Geometry check sheet. Reference: the model listing, model coordinates, mm. A direction names the side the tool comes from. Round coordinates to 2 decimals unless told otherwise and drop trailing zeros. Write each loop counter-clockwise with the first axis right and the second up, starting at its lowest first coordinate (ties: lowest second). Pieces come first, ordered by that corner, then holes. Notation, with made-up numbers: (13.5, 71) - (36.5, 71) arc R8 cw to (36.5, 81) - close; hole circle Ø9 at (71.5, -22). An arc over 180 degrees is marked (long way). One line per question, with ' | ' between items. Start each with the question number.
from build123d import *

# Parameters (mm, degrees)
EXTRUDE_1_DEPTH           = 7
SKETCH_6_R                = 7
EXTRUDE_5_DEPTH           = 13
SKETCH_8_R                = 2
CUT_EXTRUDE_2_DEPTH       = 30
SKETCH_9_R                = 5
CUT_EXTRUDE_3_DEPTH       = 2.65
CUT_EXTRUDE_START         = -2.65
SKETCH_10_R               = 5
CUT_EXTRUDE_4_DEPTH       = 2.65
HOLE_WIZARD_2_D           = 3.5
HOLE_WIZARD_2_DEPTH       = 20
HOLE_WIZARD_2_CBORE_D     = 6.5
HOLE_WIZARD_2_CBORE_DEPTH = 3.1
HOLE_WIZARD_2_TIP         = 1.051506083


with BuildPart() as part:
    # 草图1 → 凸台-拉伸1 (new body)
    with BuildSketch(Plane(origin=(0, 0, 0), x_dir=(1, 0, 0), z_dir=(0, 1, 0))):
        with BuildLine():
            Line((9.486832981, -13.5), (-9.486832981, -13.5))
            ThreePointArc((-9.486832981, -13.5), (-11.66726189, -11.66726189), (-13.5, -9.486832981))
            Line((-13.5, -9.486832981), (-13.5, 9.486832981))
            ThreePointArc((-13.5, 9.486832981), (-11.66726189, 11.66726189), (-9.486832981, 13.5))
            Line((-9.486832981, 13.5), (9.486832981, 13.5))
            ThreePointArc((9.486832981, 13.5), (11.66726189, 11.66726189), (13.5, 9.486832981))
            Line((13.5, 9.486832981), (13.5, -9.486832981))
            ThreePointArc((13.5, -9.486832981), (11.66726189, -11.66726189), (9.486832981, -13.5))
        make_face()
    extrude(amount=EXTRUDE_1_DEPTH)

    # 草图6 → 凸台-拉伸5 (add)
    with BuildSketch(Plane(origin=(0, 7, 0), x_dir=(1, 0, 0), z_dir=(0, 1, 0))):
        with Locations(Location((0, 0, 0), (0, 0, 90))):
            Circle(SKETCH_6_R)
    extrude(amount=EXTRUDE_5_DEPTH)

    # 草图8 → 切除-拉伸2 (cut)
    with BuildSketch(Plane(origin=(0, 20, 0), x_dir=(1, 0, 0), z_dir=(0, 1, 0))):
        with Locations(Location((0, 0, 0), (0, 0, 270))):
            Circle(SKETCH_8_R)
    extrude(amount=-CUT_EXTRUDE_2_DEPTH, mode=Mode.SUBTRACT)

    # 草图9 → 切除-拉伸3 (cut)
    with BuildSketch(Plane(origin=(0, 20, 0), x_dir=(1, 0, 0), z_dir=(0, 1, 0))):
        with Locations(Location((0, 0, 0), (0, 0, 270))):
            Circle(SKETCH_9_R)
    extrude(amount=-CUT_EXTRUDE_3_DEPTH, mode=Mode.SUBTRACT)

    # 草图10 → 切除-拉伸4 (cut)
    with BuildSketch(Plane.XZ.offset(CUT_EXTRUDE_START)):
        with Locations(Location((0, 0, 0), (0, 0, 90))):
            Circle(SKETCH_10_R)
    extrude(amount=CUT_EXTRUDE_4_DEPTH, mode=Mode.SUBTRACT)

    # 孔2
    with Locations(Plane(origin=(0, 0, 0), x_dir=(-1, 0, 0), z_dir=(0, -1, 0))):
        with Locations((-8.209852454, 8.492066132), (8.626364404, 8.339687642), (8.471576116, -8.762786544), (-8.626364404, -8.339687642)):
            CounterBoreHole(HOLE_WIZARD_2_D / 2, HOLE_WIZARD_2_CBORE_D / 2, HOLE_WIZARD_2_CBORE_DEPTH, depth=HOLE_WIZARD_2_DEPTH)
            with Locations((0, 0, -(HOLE_WIZARD_2_DEPTH + HOLE_WIZARD_2_TIP / 2))):  # 118° drill point
                Cone(0, HOLE_WIZARD_2_D / 2, HOLE_WIZARD_2_TIP, mode=Mode.SUBTRACT)


solid = part.part
Q1. Section check D-D, the plane y = 1.5. Record the cut outline in (x, z), then the cut area to 3 significant figures.
Q2. Go/stop test with flat-tipped pins: P1, Ø3, axis at x = 1, z = 0, coming from the -Y side; P2, Ø6.5, axis at x = 0, z = 0, coming from the +Y side; P3, Ø4, axis at x = 8.21, z = -8.49, coming from the -Y side. Record where each tip stops, or that it passes through.
Q3. Section check C-C, the plane x = 9. Record the cut outline in (y, z).
Q4. Draft check along X on faces 1 (the flat face through (-0.1, 2.65, 2.2)), 2 (the cylindrical face through (11.639, 3.451, -11.695)), 3 (the flat face through (0, 0, -6)). Enter one of: pulls with the +X half, pulls with the -X half, needs draft (parallel to the pull), parting line crosses it, or undercut.
Q5. Set-up check for faces 4 (the cylindrical face through (6.834, 13.409, 1.517)), 5 (the flat face through (-10, 3.1, 10)), 6 (the flat face through (0, 3, 13.5)): record each of +Z, -Z, +X, -X, +Y, -Y from which the full face is reachable in a straight line by a thin tool's end or side.
Q6. Section check A-A, the plane z = 0. Record the cut outline in (x, y).
Q7. Section check B-B, the plane x = 0. Record the cut outline in (y, z), then the cut area to 3 significant figures.
Q8. Thickness scan on line 1 (Z direction, x = 11, y = 2.25); line 2 (Z direction, x = 8.5, y = 3.25); line 3 (X direction, y = 0.7, z = 0). Record the ranges inside material, lowest first.
Result sheet:
1) outline: (-13.5, -9.49) arc R16.5 ccw to (-9.49, -13.5) - (9.49, -13.5) arc R16.5 ccw to (13.5, -9.49) - (13.5, 9.49) arc R16.5 ccw to (9.49, 13.5) - (-9.49, 13.5) arc R16.5 ccw to (-13.5, 9.49) - close; hole circle Ø6.5 at (-8.63, -8.34); hole circle Ø6.5 at (-8.47, 8.76); hole circle Ø10 at (0, 0); hole circle Ø6.5 at (8.21, -8.49); hole circle Ø6.5 at (8.63, 8.34) | area: 489 mm²
2) P1: y = 2.65 | P2: y = 17.35 | P3: y = 3.1
3) outline: (0, -13.5) - (7, -13.5) - (7, -10.05) - (3.1, -10.05) - (3.1, -11.64) - (0, -11.64) - close; (0, -5.34) - (3.1, -5.34) - (3.1, -6.93) - (7, -6.93) - (7, 6.63) - (3.1, 6.63) - (3.1, 5.11) - (0, 5.11) - close; (0, 11.57) - (3.1, 11.57) - (3.1, 10.05) - (7, 10.05) - (7, 13.5) - (0, 13.5) - close
4) face 1: undercut | face 2: pulls with the +X half | face 3: needs draft
5) face 4: +Y | face 5: -Y | face 6: +Z, +X, -X, +Y, -Y
6) outline: (-13.5, 0) - (-5, 0) - (-5, 2.65) - (-2, 2.65) - (-2, 17.35) - (-5, 17.35) - (-5, 20) - (-7, 20) - (-7, 7) - (-13.5, 7) - close; (2, 2.65) - (5, 2.65) - (5, 0) - (13.5, 0) - (13.5, 7) - (7, 7) - (7, 20) - (5, 20) - (5, 17.35) - (2, 17.35) - close
7) outline: (0, -13.5) - (7, -13.5) - (7, -7) - (20, -7) - (20, -5) - (17.35, -5) - (17.35, -2) - (2.65, -2) - (2.65, -5) - (0, -5) - close; (0, 5) - (2.65, 5) - (2.65, 2) - (17.35, 2) - (17.35, 5) - (20, 5) - (20, 7) - (7, 7) - (7, 13.5) - (0, 13.5) - close | area: 259 mm²
8) line 1: -12.3 to -10.16, -6.83 to 6.12, 10.56 to 12.3 | line 2: -13.5 to -10.22, -6.77 to 6.59, 10.09 to 13.5 | line 3: -13.5 to -5, 5 to 13.5
